Input: part model. Units: mm. Frame: model coordinates. A direction names the side the tool comes from. Coordinates: 2 decimals unless noted, no trailing zeros. Write each loop counter-clockwise with the first axis right and the second up, starting at its lowest first coordinate (ties: lowest second). Pieces come first, ordered by that corner, then holes.
1) Draft query along Z for faces 1 (the cylindrical face through (6.47, 1.43, 20.75)), 2 (the flat face through (3.5, 3.7, 0)), 3 (the flat face through (13, 6, 22)), 4 (the cylindrical face through (6.47, 1.43, 11.75)). Return one class per face: pulls with the +Z half, pulls with the -Z half, needs draft (parallel to the pull), parting line crosses it, or undercut.
2) Line query: L1, parallel to X at y = 11.85, z = 14; L2, parallel to Y at x = 6.75, z = 38.5; L3, parallel to Y at x = 3.5, z = 19.5. Output: solid intervals per line, ascending.
3) Pin query (flat end, axial travel): pin 1 Ø7 at (x, y) = (6.5, 6.5) entering from -Z. Return the tip coordinate at first contact, or that it passes through.
4) Set-up query: faces 5 (the flat face through (0, 7, 22)), 6 (the cylindrical face through (7.936, 9.964, 20.534)). Return all of +Z, -Z, +X, -X, +Y, -Y with unobstructed straight access to the full face (end or side cutting, diameter ignored); none if empty.
5) Section query C-C (x = 9.25). Output: boundary loops of the cut face in (y, z).
6) Section query A-A (z = 20). Output: boundary loops of the cut face in (x, y), then the cut area to 3 significant figures.
7) Section query B-B (y = 6.5). Output: boundary loops of the cut face in (x, z), then the cut area to 3 significant figures.
Autodesk Inventor part; units mm, degrees
ref_plane "YZ Plane" through (0, 0, 0) normal (1, 0, 0) x (0, 1, 0)
ref_plane "XZ Plane" through (0, 0, 0) normal (0, 1, 0) x (-1, 0, 0)
ref_plane "XY Plane" through (0, 0, 0) normal (0, 0, 1) x (1, 0, 0)
sketch "Sketch1" plane through (0, 0, 0) normal (0, 0, 1) x (1, 0, 0)
  line L0 (0, 0) -> (13, 0)
  line L1 (13, 0) -> (13, 13)
  line L2 (13, 13) -> (0, 13)
  line L3 (0, 13) -> (0, 0)
  dimension "d0" = 13
  dimension "d1" = 13
extrude "Extrusion1" add sketch "Sketch1" along normal blind 45
sketch "Sketch2" plane through (0, 0, 0) normal (0, 0, -1) x (-1, 0, 0)
  circle A0 centre (-6.5, 6.5) radius 3.75
  line L0 (0, 13) -> (0, 0)
  line L1 (0, 0) -> (-13, 0)
  dimension "d4" = 7.5
  dimension "d5" = 6.5
  dimension "d6" = 6.5
hole "Hole1" at (6.5, 6.5, 0) direction (0, 0, 1) diameter 4.5 end through all counterbore diameter 7.5 counterbore depth 40.5
sketch "Sketch3" plane through (0, 0, 0) normal (0, -1, 0) x (1, 0, 0)
  circle A0 centre (6.5, 5) radius 1
  line L0 (13, 0) -> (13, 45)
  line L1 (0, 0) -> (13, 0)
  circle A1 centre (6.5, 8) radius 1
  circle A2 centre (6.5, 11) radius 1
  circle A3 centre (6.5, 14) radius 1
  circle A4 centre (6.5, 17) radius 1
  circle A5 centre (6.5, 20) radius 1
  dimension "d14" = 2
  dimension "d15" = 6.5
  dimension "d16" = 5
  dimension "d17" = 2
  dimension "d18" = 3
  dimension "d19" = 6.5
  dimension "d20" = 2
  dimension "d21" = 3
  dimension "d22" = 6.5
  dimension "d23" = 2
  dimension "d24" = 3
  dimension "d25" = 6.5
  dimension "d26" = 2
  dimension "d27" = 3
  dimension "d28" = 2
  dimension "d29" = 3
  dimension "d30" = 6.5
hole "Hole2" at (6.5, 0, 5) at (6.5, 0, 8) at (6.5, 0, 11) at (6.5, 0, 14) at (6.5, 0, 17) at (6.5, 0, 20) direction (0, 1, 0) diameter 1.5 end through all
equation "\"d12\" = Thickness"
equation "\"d36\" = Thickness"
equation "\"BendRadius\" = Thickness"
equation "\"BendReliefWidth\" = Thickness"
equation "\"BendReliefDepth\" = 0.5 * Thickness"
equation "\"CornerReliefSize\" = 4 * Thickness"
equation "\"MinimumRemnant\" = 2 * Thickness"
equation "\"TransitionRadius\" = BendRadius"
equation "\"JacobiRadiusSize\" = BendRadius"
equation "\"GapSize\" = Thickness"
properties part number "male_long_part2_9_2018" material "Acetal Resin, Black"
Answer:
1. face 1: undercut
1. face 2: pulls with the -Z half
1. face 3: needs draft
1. face 4: undercut
2. L1: x = 0 to 5.75, 7.25 to 13
2. L2: y = 0 to 2.76, 10.24 to 13
2. L3: y = 0 to 4.25, 8.75 to 13
3. pin 1: stops at z = 40.5
4. face 5: +Z, -Z, -X, +Y, -Y
4. face 6: -Z
5. outline: (0, 0) - (3.95, 0) - (3.95, 40.5) - (9.05, 40.5) - (9.05, 0) - (13, 0) - (13, 45) - (0, 45) - close
6. outline: (0, 0) - (5.75, 0) - (5.75, 2.83) arc R3.75 cw to (5.75, 10.17) - (5.75, 13) - (0, 13) - close; (7.25, 0) - (13, 0) - (13, 13) - (7.25, 13) - (7.25, 10.17) arc R3.75 cw to (7.25, 2.83) - close
6. area: 116 mm2
7. outline: (0, 0) - (2.75, 0) - (2.75, 40.5) - (4.25, 40.5) - (4.25, 45) - (0, 45) - close; (8.75, 40.5) - (10.25, 40.5) - (10.25, 0) - (13, 0) - (13, 45) - (8.75, 45) - close
7. area: 261 mm2
